Build history of the part. All positions in model axes, mm. Face numbers are marked on the shaded views. A direction names the side the tool comes from. Round coordinates to 2 decimals unless told otherwise and drop trailing zeros. Loops run counter-clockwise (first coordinate to the right, second up) from the corner with the lowest first, then second, coordinate; pieces in that order, holes last.
from build123d import *

# Parameters (mm, degrees)
SKETCH1_W                 = 49
SKETCH1_H                 = 49
BOSS_EXTRUDE1_DEPTH       = 4.5
SKETCH3_W                 = 42
SKETCH3_H                 = 42
BOSS_EXTRUDE3_DEPTH       = 5.5
SKETCH4_W                 = 11
SKETCH4_H                 = 10
SKETCH4_W_2               = 10
SKETCH4_H_2               = 11
BOSS_EXTRUDE5_DEPTH       = 15
F_3_0MM_DOWEL_SLOT1_D     = 3
F_3_0MM_DOWEL_SLOT2_D     = 3
SKETCH15_W                = 15
SKETCH15_H                = 2
BOSS_EXTRUDE7_DEPTH       = 3.5
BOSS_EXTRUDE7_DEPTH_BACK  = 13.5
F_3_0MM_DOWEL_SLOT3_D     = 3
SKETCH18_W                = 15
SKETCH18_H                = 2
BOSS_EXTRUDE8_DEPTH       = 3.5
BOSS_EXTRUDE8_DEPTH_BACK  = 13.5
F_3_0MM_DOWEL_SLOT5_D     = 3
SKETCH23_W                = 15
SKETCH23_H                = 2
BOSS_EXTRUDE9_DEPTH       = 3.5
BOSS_EXTRUDE9_DEPTH_BACK  = 13.5
SKETCH24_W                = 15
SKETCH24_H                = 2
BOSS_EXTRUDE10_DEPTH      = 3.5
BOSS_EXTRUDE10_DEPTH_BACK = 13.5
F_3_0MM_DOWEL_SLOT6_D     = 3


with BuildPart() as part:
    # Sketch1 → Boss-Extrude1 (new body)
    with BuildSketch(Plane(origin=(0, 0, 0), x_dir=(0, 0, -1), z_dir=(1, 0, 0))):
        Rectangle(SKETCH1_W, SKETCH1_H)
    extrude(amount=BOSS_EXTRUDE1_DEPTH)

    # Sketch3 → Boss-Extrude3 (add)
    with BuildSketch(Plane(origin=(4.5, 0, 0), x_dir=(0, 0, -1), z_dir=(1, 0, 0))):
        Rectangle(SKETCH3_W, SKETCH3_H)
    extrude(amount=BOSS_EXTRUDE3_DEPTH)

    # Sketch4 → Boss-Extrude5 (add)
    with BuildSketch(Plane(origin=(10, 0, 0), x_dir=(0, 0, -1), z_dir=(1, 0, 0))):
        with Locations((14.5, 0)):
            Rectangle(SKETCH4_W, SKETCH4_H)
        with Locations((0, -14.5)):
            Rectangle(SKETCH4_W_2, SKETCH4_H_2)
        with Locations((-14.5, 0)):
            Rectangle(SKETCH4_W, SKETCH4_H)
        with Locations((0, 14.5)):
            Rectangle(SKETCH4_W_2, SKETCH4_H_2)
    extrude(amount=BOSS_EXTRUDE5_DEPTH)

    # Ø3.0mm Dowel Slot1 (through all)
    with Locations(Plane(origin=(0, 0, -20), x_dir=(-1, 0, 0), z_dir=(0, 0, -1))):
        with Locations((-17.558984138, 0)):
            Hole(F_3_0MM_DOWEL_SLOT1_D / 2)

    # Ø3.0mm Dowel Slot2 (through all)
    with Locations(Plane(origin=(0, 20, 0), x_dir=(1, 0, 0), z_dir=(0, 1, 0))):
        with Locations((17.80910446, 0)):
            Hole(F_3_0MM_DOWEL_SLOT2_D / 2)

    # Sketch15 → Boss-Extrude7 (add, two sides)
    with BuildSketch(Plane.XY.offset(5)) as boss_extrude7_sk:
        with Locations((17.5, -11.9)):
            Rectangle(SKETCH15_W, SKETCH15_H)
    extrude(amount=BOSS_EXTRUDE7_DEPTH)
    extrude(boss_extrude7_sk.sketch, amount=-BOSS_EXTRUDE7_DEPTH_BACK)

    # Ø3.0mm Dowel Slot3 (through all)
    with Locations(Plane(origin=(17.80910446, -20, 0), x_dir=(0, 0, -1), z_dir=(0, -1, 0))):
        with Locations((0, 0)):
            Hole(F_3_0MM_DOWEL_SLOT3_D / 2)

    # Sketch18 → Boss-Extrude8 (add, two sides)
    with BuildSketch(Plane(origin=(0, 0, -5), x_dir=(-1, 0, 0), z_dir=(0, 0, -1))) as boss_extrude8_sk:
        with Locations((-17.5, 11.5)):
            Rectangle(SKETCH18_W, SKETCH18_H)
    extrude(amount=BOSS_EXTRUDE8_DEPTH)
    extrude(boss_extrude8_sk.sketch, amount=-BOSS_EXTRUDE8_DEPTH_BACK)

    # Ø3.0mm Dowel Slot5 (through all)
    with Locations(Plane(origin=(0, 20, 0), x_dir=(1, 0, 0), z_dir=(0, 1, 0))):
        with Locations((17.80910446, 0)):
            Hole(F_3_0MM_DOWEL_SLOT5_D / 2)

    # Sketch23 → Boss-Extrude9 (add, two sides)
    with BuildSketch(Plane.XZ.offset(5)) as boss_extrude9_sk:
        with Locations((17.5, -11.5)):
            Rectangle(SKETCH23_W, SKETCH23_H)
    extrude(amount=BOSS_EXTRUDE9_DEPTH)
    extrude(boss_extrude9_sk.sketch, amount=-BOSS_EXTRUDE9_DEPTH_BACK)

    # Sketch24 → Boss-Extrude10 (add, two sides)
    with BuildSketch(Plane.XZ.offset(5)) as boss_extrude10_sk:
        with Locations((17.5, 11.5)):
            Rectangle(SKETCH24_W, SKETCH24_H)
    extrude(amount=BOSS_EXTRUDE10_DEPTH)
    extrude(boss_extrude10_sk.sketch, amount=-BOSS_EXTRUDE10_DEPTH_BACK)

    # Ø3.0mm Dowel Slot6 (through all)
    with Locations(Plane.XY.offset(20)):
        with Locations((17.558984138, 0)):
            Hole(F_3_0MM_DOWEL_SLOT6_D / 2)


solid = part.part
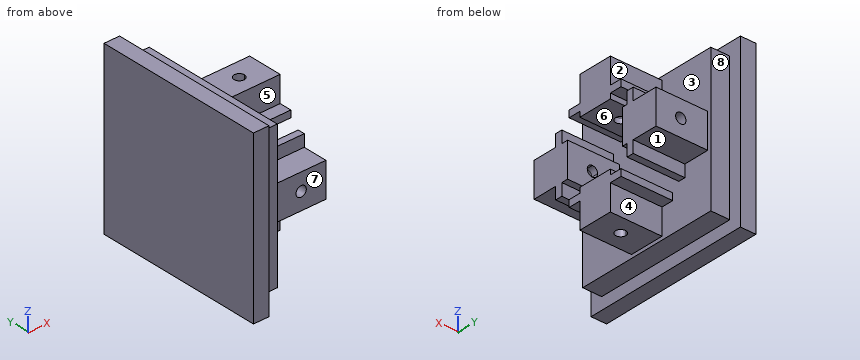
(1) Which spindle directions (+Z, -Z, +X, -X, +Y, -Y) get a long thin tool onto all of the face, cutting with end or side? Do the marked faces 4, 5, 6, 7 and 8. Say none if no direction does.
Responses:
face 4: -Z, +X, +Y
face 5: +Z, +X, -Y
face 6: +X, +Y, -Y
face 7: +Z, -Z, +X, -Y
face 8: +Z, -Z, +X, +Y
(2) Pull direction Z, two halves, no side cores. Call the marked faces 1, 2 and 3: +Z half, -Z half, draft (parallel to the pull), parting line (faces both ways), or undercut.
Responses:
face 1: -Z half
face 2: draft
face 3: undercut
(3) Slice it at C-C on y = -3. List the corners of the cut face in (x, z), plus the area to 4 significant figures.
Responses:
outline: (0, -24.5) - (4.5, -24.5) - (4.5, -21) - (10, -21) - (10, -20) - (25, -20) - (25, -9) - (10, -9) - (10, 9) - (25, 9) - (25, 20) - (10, 20) - (10, 21) - (4.5, 21) - (4.5, 24.5) - (0, 24.5) - close
area: 781.5 mm2
(4) Pin check, flat tips, straight feed: P1, Ø5, axis at x = 20.5, z = 0, coming from the +Y side; P2, Ø12, axis at x = 17, y = -10.5, coming from the -Z side; P3, Ø8, axis at x = 20.5, z = -17.5, coming from the -Y side. Stop position of each tip, or through.
Responses:
P1: stops at y = 20
P2: stops at z = -20
P3: stops at y = -5
(5) Slice it at B-B on z = 15. List the corners of the cut face in (x, y).
Responses:
outline: (0, -24.5) - (4.5, -24.5) - (4.5, -21) - (10, -21) - (10, -5) - (25, -5) - (25, 5) - (10, 5) - (10, 21) - (4.5, 21) - (4.5, 24.5) - (0, 24.5) - close; hole circle Ø3 at (17.56, 0)
(6) Probe line 1 (Z direction, x = 17.5, y = -2); line 2 (Y direction, x = 21, z = -5.5); line 3 (Z direction, x = 17, y = 5.5). List the from-to ranges inside material, lowest first.
Responses:
line 1: z = -20 to -9, 9 to 20
line 2: y = -12.9 to -10.9, 10.5 to 12.5
line 3: z = -12.5 to -10.5, 10.5 to 12.5
(7) Slice it at D-D on z = -7. List the corners of the cut face in (x, y).
Responses:
outline: (0, -24.5) - (4.5, -24.5) - (4.5, -21) - (10, -21) - (10, -12.9) - (25, -12.9) - (25, -10.9) - (10, -10.9) - (10, 10.5) - (25, 10.5) - (25, 12.5) - (10, 12.5) - (10, 21) - (4.5, 21) - (4.5, 24.5) - (0, 24.5) - close
(8) Slice it at A-A on y = 16. List the corners of the cut face in (x, z), plus the area to 3 significant figures.
Responses:
outline: (0, -24.5) - (4.5, -24.5) - (4.5, -21) - (10, -21) - (10, -5) - (25, -5) - (25, 5) - (10, 5) - (10, 21) - (4.5, 21) - (4.5, 24.5) - (0, 24.5) - close; hole circle Ø3 at (17.81, 0)
area: 594 mm2
